Autodesk Inventor part; units mm, degrees
ref_plane "YZ Plane" through (0, 0, 0) normal (1, 0, 0) x (0, 1, 0)
ref_plane "XZ Plane" through (0, 0, 0) normal (0, 1, 0) x (-1, 0, 0)
ref_plane "XY Plane" through (0, 0, 0) normal (0, 0, 1) x (1, 0, 0)
sketch "スケッチ1" plane through (0, 0, 0) normal (0, 1, 0) x (-1, 0, 0)
  line L0 (0, 0) -> (-70, 0)
  line L1 (-70, 0) -> (-70, 10)
  line L2 (-70, 10) -> (0, 10)
  line L3 (0, 10) -> (0, 0)
  dimension "d0" = 70
  dimension "d1" = 10
extrude "押し出し1" add sketch "スケッチ1" along normal blind 10
sketch "スケッチ17" plane through (0, 10, 0) normal (0, 1, 0) x (1, 0, 0)
  line L0 (70, 0) -> (0, 0)
  line L1 (0, 0) -> (0, -10)
  line L2 (0, -10) -> (70, -10)
  line L3 (0, -5) -> (4.5, -5)
  line L4 (4.5, -5) -> (4.5, 0)
  line L5 (70, -5) -> (65.5, -5)
  point P0 (7.0002, -10)
  point P1 (7.0002, 0)
  dimension "d42" = 4.5
  dimension "d43" = 5
  dimension "d44" = 4.5
  dimension "d52" = 61
hole "穴1" at (4.5, 10, 5) at (65.5, 10, 5) direction (0, -1, 0) diameter 3 depth 10 tip angle 118
sketch "スケッチ18" plane through (70, 0, 0) normal (0, 0, -1) x (-1, 0, 0)
  line L0 (70, 0) -> (0, 0)
  line L1 (0, 10) -> (70, 10)
  line L2 (0, 10) -> (2, 10)
  line L3 (2, 10) -> (2, 0)
  line L4 (2, 0) -> (0, 0)
  line L5 (0, 0) -> (0, 10)
  line L6 (70, 0) -> (68, 0)
  line L7 (68, 0) -> (68, 10)
  line L8 (68, 10) -> (70, 10)
  line L9 (70, 10) -> (70, 0)
  point P0 (62.9998, 10)
  dimension "d53" = 2
  dimension "d54" = 2
extrude "押し出し15" cut sketch "スケッチ18" against normal blind 10 contours L0 L7 L1 L9 | L0 L5 L1 L3
sketch "スケッチ19" plane through (0, 10, 0) normal (0, 1, 0) x (1, 0, 0)
  line L0 (68, 0) -> (2, 0)
  line L1 (2, -10) -> (68, -10)
  line L2 (7.4699, 0) -> (62.4699, 0)
  line L3 (62.4699, 0) -> (62.4699, -10)
  line L4 (62.4699, -10) -> (7.4699, -10)
  line L5 (7.4699, -10) -> (7.4699, 0)
  point P0 (0, 0)
  dimension "d57" = 55
extrude "押し出し16" add sketch "スケッチ19" along normal blind 1
properties part number "知能ロボコンラックギア" material "鋼、炭素鋼"
Input: part model. Units: mm. Frame: model coordinates. A direction names the side the tool comes from. Give positions to 0.01 mm unless a question says otherwise; leave off trailing zeros. Order: outer loops, then holes, each group sorted by start corner. A loop starts at its lowest first (then second) coordinate and runs counter-clockwise, first axis right, second up. Notation, with made-up numbers: (44, 48) -> (56, 48) arc R19 cw to (56, 84) -> close; hole circle Ø4 at (11.25, -39.5). An arc over 180 degrees is marked (long way). Use one line per item in the form item = value.
1) Section A-A, the plane z = 5. Return loops of the section in (x, y), and give its area (3 significant figures).
Response values:
outline = (2, 0) -> (3, 0) -> (3, 10) -> (2, 10) -> close; (6, 0) -> (64, 0) -> (64, 10) -> (62.47, 10) -> (62.47, 11) -> (7.47, 11) -> (7.47, 10) -> (6, 10) -> close; (67, 0) -> (68, 0) -> (68, 10) -> (67, 10) -> close
area = 655 mm^2
2) Section B-B, the plane x = 4.5. Return loops of the section in (y, z).
Response values:
outline = (0, 0) -> (10, 0) -> (10, 3.5) -> (0, 3.5) -> close; (0, 6.5) -> (10, 6.5) -> (10, 10) -> (0, 10) -> close
3) Section C-C, the plane y = 3. Return loops of the section in (x, z), and give its area (3 significant figures).
Response values:
outline = (2, 0) -> (68, 0) -> (68, 10) -> (2, 10) -> close; hole circle Ø3 at (4.5, 5); hole circle Ø3 at (65.5, 5)
area = 646 mm^2
4) Reachability of faces 4 (the flat face through (64, 10, 6)), 5 (the flat face through (35, 5, 10)), 6 (the flat face through (6, 10, 6)) from +Z, -Z, +X, -X, +Y, -Y: full face, straight path, thin tool, end or side. Return the list, or none.
Response values:
face_4 = +Z, -Z, +X, +Y
face_5 = +Z, +X, -X, +Y, -Y
face_6 = +Z, -Z, -X, +Y
5) First-contact query: pin 1 Ø2.5 at (x, z) = (3.5, 4.5) entering from +Y. Flat tip, straight axial feed; report the tip coordinate or a pass-through.
Response values:
pin_1 = 10
6) Mould query, pull axis X, two halves, no side actions, for faces 1 (the flat face through (35, 11, 5)), 2 (the flat face through (2, 5, 5)), 3 (the cylindrical face through (3.235, 4.93, 5.806)). Classes: pulls with the +X half, pulls with the -X half, needs draft (parallel to the pull), parting line crosses it, or undercut.
Response values:
face_1 = needs draft
face_2 = pulls with the -X half
face_3 = undercut
7) Line query: probe 1 along X at (y, z) = (5.25, 5); probe 2 along X at (y, z) = (8.5, 3.75); probe 3 along Z at (x, y) = (4.5, 4.5). Output: solid intervals per line, ascending.
Response values:
probe_1 = 2 to 3, 6 to 64, 67 to 68
probe_2 = 2 to 3.67, 5.33 to 64.67, 66.33 to 68
probe_3 = 0 to 3.5, 6.5 to 10
